Solid Edge part; units mm, degrees
sketch "Sketch1" plane through (0, 0, 0) normal (0, 0, 1) x (1, 0, 0)
  line L0 (0, 0) -> (0, 31.75)
  line L1 (0, 31.75) -> (76.2, 31.75)
  line L2 (76.2, 31.75) -> (76.2, 0)
  line L3 (76.2, 0) -> (0, 0)
  dimension "D1" = 76.2
extrude "Protrusion1" add sketch "Sketch1" along normal blind 3.175
hole "Hole_1" at (38.1, 23.8125, 3.175) direction (0, 0, -1) diameter 6.7564 end up to next
hole "Hole1" at (66.675, 23.8125, 3.175) direction (0, 0, -1) diameter 6.7564 end up to next
hole "Hole2" at (9.525, 23.8125, 3.175) direction (0, 0, -1) diameter 6.7564 end up to next
hole "Hole3" at (66.675, 6.35, 3.175) direction (0, 0, -1) diameter 4.826 end up to next countersink diameter 10.287 countersink angle 82
hole "Hole4" at (9.525, 6.35, 3.175) direction (0, 0, -1) diameter 4.826 end up to next countersink diameter 10.287 countersink angle 82
The model under review builds one solid part; all positions refer to its coordinate system, in mm. Round coordinates to 2 decimals unless told otherwise and drop trailing zeros. Write each loop counter-clockwise with the first axis right and the second up, starting at its lowest first coordinate (ties: lowest second). Pieces come first, ordered by that corner, then holes.
(1) We need section D-D on y = 26. Give the boundary of the cut face in (x, z) (3 decimals).
(2) Insertion check: pin 1 (4 mm diameter, centred on x = 66.68, y = 23.81, fed in from +Z). The pin has a flat end and moves straight along its axis. Give the tip position at first contact, or say it passes through.
(3) We need section B-B on x = 38.1. Give the boundary of the cut face in (y, z) (3 decimals), and give its area (3 significant figures).
(4) Wall thickness on L1, parallel to X at y = 6.35, z = 0.05; L2, parallel to X at y = 22.5, z = 1.9; L3, parallel to Y at x = 64.5, z = 1.3: over which ranges is each line inside the solid? List them lowest first.
(5) Mouldability with a two-part tool opening along X and no side actions: class faces 1 (the flat face through (0, 16, 2)), 2 (the flat face through (38, 31.75, 2)), 3 (the flat face through (76.2, 16, 2)), 4 (the cylindrical face through (10.54, 20.59, 1.61)) as +X half, -X half, draft (parallel to the pull), parting line (faces both ways), or undercut.
(6) We need section A-A on y = 6.35. Give the number of separate pieces and of enclosed holes in the cut face, and give its area (3 significant figures).
Findings below:
1. outline: (0, 0) - (6.951, 0) - (6.951, 3.175) - (0, 3.175) - close; (12.099, 0) - (35.526, 0) - (35.526, 3.175) - (12.099, 3.175) - close; (40.674, 0) - (64.101, 0) - (64.101, 3.175) - (40.674, 3.175) - close; (69.249, 0) - (76.2, 0) - (76.2, 3.175) - (69.249, 3.175) - close
2. pin 1: passes through
3. outline: (0, 0) - (20.434, 0) - (20.434, 3.175) - (0, 3.175) - close; (27.191, 0) - (31.75, 0) - (31.75, 3.175) - (27.191, 3.175) - close
3. area: 79.4 mm2
4. L1: x = 0 to 7.1, 11.95 to 64.25, 69.1 to 76.2
4. L2: x = 0 to 6.41, 12.64 to 34.99, 41.21 to 63.56, 69.79 to 76.2
4. L3: y = 0 to 3.59, 9.11 to 21.23, 26.4 to 31.75
5. face 1: -X half
5. face 2: draft
5. face 3: +X half
5. face 4: undercut
6. separate pieces: 3
6. enclosed holes: 0
6. area: 194 mm2
